Build history of the part. All positions in model axes, mm. Round coordinates to 2 decimals unless told otherwise and drop trailing zeros. Write each loop counter-clockwise with the first axis right and the second up, starting at its lowest first coordinate (ties: lowest second). Pieces come first, ordered by that corner, then holes. Notation, with made-up numbers: (8, 11.25) -> (58, 11.25) arc R28 ccw to (58, 46.25) -> close; hole circle Ø6 at (87, 64.5). An arc over 180 degrees is marked (long way). One line per question, with ' | ' between items.
from build123d import *

# Parameters (mm, degrees)
F0_W     = 50.8
F0_H     = 50.8
F1_DEPTH = 12.7
F2_W     = 50.8
F2_H     = 50.8
F2_R     = 17.4625
F3_DEPTH = 25.4


with BuildPart() as f1:
    # F0 (on Top) → F1 (new body, symmetric)
    with BuildSketch(Plane.XY):
        Rectangle(F0_W, F0_H)
    extrude(amount=F1_DEPTH, both=True)

    # F2 (on face) → F3 (intersect, through all)
    with BuildSketch(Plane.XY.offset(12.7)):
        Rectangle(F2_W, F2_H)
        Circle(F2_R, mode=Mode.SUBTRACT)
    extrude(amount=-F3_DEPTH, mode=Mode.INTERSECT)


solid = f1.part
(1) Drop a flat-ended pin along its axis: pin 1 (21 mm diameter, centred on x = 0, y = 0, fed in from -Z). Give the stop position or say it passes through.
Calculated:
pin 1: through
(2) Mould opens along Y. For faces 1 (the cylindrical face through (-13.858, -10.626, 0.178)), 2 (the flat face through (-25.4, 0, 0)), 3 (the flat face through (0, -25.4, 0)) say: pulls with the +Y half, pulls with the -Y half, needs draft (parallel to the pull), parting line crosses it, or undercut.
Calculated:
face 1: undercut | face 2: needs draft | face 3: pulls with the -Y half
(3) Slice it at A-A (x = 0). Write the cut outline in (y, z), then the cut area to 3 significant figures.
Calculated:
outline: (-25.4, -12.7) -> (-17.46, -12.7) -> (-17.46, 12.7) -> (-25.4, 12.7) -> close; (17.46, -12.7) -> (25.4, -12.7) -> (25.4, 12.7) -> (17.46, 12.7) -> close | area: 403 mm2
(4) Slice it at C-C (z = -4.25). Write the cut outline in (x, y) (1 decimal), then the cut area to 3 significant figures.
Calculated:
outline: (-25.4, -25.4) -> (25.4, -25.4) -> (25.4, 25.4) -> (-25.4, 25.4) -> close; hole circle Ø34.9 at (0, 0) | area: 1,620 mm2
(5) Wall check: line 1 (Y direction, x = 0, z = 3.75); line 2 (Y direction, x = -11.5, z = 1); line 3 (X direction, y = -2, z = 2). Give the ranges that are in metal, low to high. Write a range as from..to.
Calculated:
line 1: -25.4..-17.46, 17.46..25.4 | line 2: -25.4..-13.14, 13.14..25.4 | line 3: -25.4..-17.35, 17.35..25.4
